For this review, take the finished solid that the model builds, in its own axes (mm). A direction names the side the tool comes from. Coordinates: 2 decimals unless noted, no trailing zeros. Loops run counter-clockwise (first coordinate to the right, second up) from the corner with the lowest first, then second, coordinate; pieces in that order, holes last.
1. Take a section at C-C, the plane x = 0. State the section outline as (y, z) points, then the cut area to 3 significant figures.
2. Take a section at A-A, the plane x = -37.5. State the section outline as (y, z) points, then the cut area to 3 significant figures.
3. To check wall thickness, follow probe 1 along X at (y, z) = (-35.5, 16.5); probe 2 along X at (y, z) = (-24.5, 31); probe 3 along X at (y, z) = (-34, 9). State the ranges of each line that lie inside material, in increasing order.
4. Mouldability with a two-part tool opening along Y and no side actions: class faces 1 (the face through (17, -38, 52.7)), 2 (the face through (-15.788, -17.696, 3.131)), 3 (the face through (17.49, -34.27, 13.36)), 4 (the face through (-39.359, -26.527, 29.569)) as pulls with the +Y half, pulls with the -Y half, needs draft (parallel to the pull), parting line crosses it, or undercut.
5. Take a section at D-D, the plane x = -15.5. State the section outline as (y, z) points, then the cut area to 3 significant figures.
6. Take a section at B-B, the plane y = -24.5. State the section outline as (x, z) points, then the cut area to 3 significant figures.
7. Machinability: for faces 5 (the face through (21.004, -10, 14)), 6 (the face through (15, -34.5, 40)), 7 (the face through (17, -40.85, 39)), 8 (the face through (-7, -27.5, 17)), which of the approach directions +Z, -Z, +X, -X, +Y, -Y give a long, thin tool a straight path to every point of the face, cutting with its end or side? Answer none if there is none.
8. Clearance check with flat-ended pins moving along their axes: P1, Ø6, axis at x = 9.5, z = 25.5, coming from the -Y side; P2, Ø5, axis at x = -21, y = -9, coming from the +Z side; P3, Ø1.5, axis at y = -13, z = 13, coming from the -X side. State where each tip first meets the part, or that it passes through.
Autodesk Inventor part; units mm, degrees
ref_plane "Work Plane1" through (0, -21.15, 0) normal (-1, 0, 0) x (0, 0, 1)
ref_plane "Work Plane2" through (-27.5, -34.5, 33.95) normal (0, -1, 0) x (1, 0, 0)
ref_plane "Work Plane3" through (-33.9, -14.5, 32.7) normal (0, 0, -1) x (0, 1, 0)
sketch "Sketch1" plane through (0, 0, 0) normal (0, 0, 1) x (1, 0, 0)
  line L0 (-21.15, 16.8267) -> (-21.15, -16.8267)
  arc A0 (-21.15, -16.8267) -> (-21.0036, -17.1802) centre (-20.65, -16.8267) ccw
  line L1 (-21.0036, -17.1802) -> (-17.1802, -21.0036)
  arc A1 (-17.1802, -21.0036) -> (-16.8267, -21.15) centre (-16.8267, -20.65) ccw
  line L2 (-16.8267, -21.15) -> (16.8267, -21.15)
  arc A2 (16.8267, -21.15) -> (17.1802, -21.0036) centre (16.8267, -20.65) ccw
  line L3 (17.1802, -21.0036) -> (21.0036, -17.1802)
  arc A3 (21.0036, -17.1802) -> (21.15, -16.8267) centre (20.65, -16.8267) ccw
  line L4 (21.15, -16.8267) -> (21.15, 16.8267)
  arc A4 (21.15, 16.8267) -> (21.0036, 17.1802) centre (20.65, 16.8267) ccw
  line L5 (21.0036, 17.1802) -> (17.1802, 21.0036)
  arc A5 (17.1802, 21.0036) -> (16.8267, 21.15) centre (16.8267, 20.65) ccw
  line L6 (16.8267, 21.15) -> (-16.8267, 21.15)
  arc A6 (-16.8267, 21.15) -> (-17.1802, 21.0036) centre (-16.8267, 20.65) ccw
  line L7 (-17.1802, 21.0036) -> (-21.0036, 17.1802)
  arc A7 (-21.0036, 17.1802) -> (-21.15, 16.8267) centre (-20.65, 16.8267) ccw
  circle A8 centre (-15.5, -15.5) radius 1.75
  circle A9 centre (-15.5, 15.5) radius 1.75
  circle A10 centre (15.5, 15.5) radius 1.75
  circle A11 centre (15.5, -15.5) radius 1.75
  circle A12 centre (0, 0) radius 17
  circle A13 centre (15.5, 15.5) radius 2.2144
  circle A14 centre (15.5, -15.5) radius 2.2144
  circle A15 centre (-15.5, -15.5) radius 2.2144
  circle A16 centre (-15.5, 15.5) radius 2.2144
  circle A17 centre (0, 0) radius 17.7962
extrude "Extrusion1" add sketch "Sketch1" along normal blind 6.35 contours A7 L7 A6 L6 A5 L5 A4 L4 A3 L3 A2 L2 A1 L1 A0 L0
sketch "Sketch2" plane through (-16.8267, -21.15, 0) normal (0, -1, 0) x (1, 0, 0)
  line L0 (0, 0) -> (33.6533, 0)
  line L1 (33.6533, 0) -> (33.6533, 6.35)
  line L2 (0, 6.35) -> (33.6533, 6.35)
  line L3 (0, 0) -> (0, 6.35)
  line L4 (-10.6733, 32.7) -> (65.5267, 32.7)
  line L5 (65.5267, 33.95) -> (-10.6733, 33.95)
  line L6 (65.5267, 33.95) -> (65.5267, 39.1)
  line L7 (65.5267, 39.1) -> (-10.6733, 39.1)
  line L8 (-10.6733, 33.95) -> (-10.6733, 39.1)
  line L9 (0, 0) -> (33.6533, 0)
  line L10 (33.6533, 0) -> (33.6533, 32.7)
  line L11 (33.6533, 32.7) -> (0, 32.7)
  line L12 (0, 32.7) -> (0, 0)
  line L13 (-4.1769, 0) -> (-0.3536, 0)
  line L14 (-0.3536, 0) -> (-0.3536, 6.35)
  line L15 (-4.1769, 6.35) -> (-0.3536, 6.35)
  line L16 (-4.1769, 0) -> (-4.1769, 6.35)
  line L17 (34.0069, 0) -> (37.8302, 0)
  line L18 (37.8302, 0) -> (37.8302, 6.35)
  line L19 (34.0069, 6.35) -> (37.8302, 6.35)
  line L20 (34.0069, 0) -> (34.0069, 6.35)
  line L21 (-4.1769, 0) -> (37.8302, 0)
  line L22 (37.8302, 0) -> (37.8302, 32.7)
  line L23 (37.8302, 32.7) -> (-4.1769, 32.7)
  line L24 (-4.1769, 32.7) -> (-4.1769, 0)
  point P0 (16.8267, 0)
extrude "Extrusion2" add sketch "Sketch2" along normal blind 6.35 contours L3 L2 L1 L0 | L21 L14 L15 L24 L4 L12 L3 | L1 L10 L4 L22 L19 L20 L21 | L12 L4 L10 L2 | L13 L16 L15 L14 | L20 L19 L18 L17
ref_plane "Work Plane1" through (0, -21.15, 0) normal (-1, 0, 0) x (0, 0, 1)
sketch "Sketch4" plane through (-21.0036, -21.15, 0) normal (-1, 0, 0) x (0, 0, 1)
  line L0 (0, 37.9767) -> (0, 4.3233)
  line L1 (0, 4.3233) -> (6.35, 4.3233)
  line L2 (6.35, 37.9767) -> (6.35, 4.3233)
  line L3 (0, 37.9767) -> (6.35, 37.9767)
  line L4 (32.7, 0) -> (0, 0)
  line L5 (0, 0) -> (0, -6.35)
  line L6 (32.7, -6.35) -> (0, -6.35)
  line L7 (32.7, 0) -> (32.7, -6.35)
  line L8 (6.35, 37.9767) -> (6.35, 4.3233)
  line L9 (32.7, 0) -> (32.7, -6.35)
  line L10 (0, 0.1464) -> (6.35, 0.1464)
  line L11 (0, 38.3302) -> (6.35, 38.3302)
  line L12 (0, 38.3302) -> (6.35, 38.3302)
  line L13 (6.35, 38.9462) -> (6.35, 3.3538)
  line L14 (6.35, 38.3302) -> (32.7, 0)
  line L15 (0, 0) -> (0, -6.35)
  line L16 (32.7, 0) -> (0, 0)
  line L17 (0, 0) -> (0, 38.3302)
  point P0 (0, 21.15)
extrude "Extrusion3" add sketch "Sketch4" along normal blind 6.35
mirror "Mirror1" about plane through (0, -21.15, 0) normal (-1, 0, 0) of "Extrusion3"
sketch "Sketch5" plane through (-16.8267, -27.5, 0) normal (0, -1, 0) x (1, 0, 0)
  line L0 (2.5767, 45.45) -> (8.0767, 45.45)
  arc A0 (8.0767, 39.95) -> (8.0767, 45.45) centre (8.0767, 42.7) ccw
  line L1 (8.0767, 39.95) -> (2.5767, 39.95)
  arc A1 (2.5767, 45.45) -> (2.5767, 39.95) centre (2.5767, 42.7) ccw
  line L2 (17.3267, 50.7) -> (-6.6733, 50.7)
  line L3 (-6.6733, 50.7) -> (-6.6733, 34.7)
  line L4 (-6.6733, 34.7) -> (17.3267, 34.7)
  line L5 (17.3267, 34.7) -> (17.3267, 50.7)
  line L6 (-10.5269, 32.7) -> (44.1802, 32.7)
  line L7 (-10.5269, 0) -> (-10.5269, 32.7)
  line L8 (44.1802, 0) -> (-10.5269, 0)
  line L9 (44.1802, 0) -> (44.1802, 32.7)
  line L10 (37.8302, 32.7) -> (44.1802, 32.7)
  line L11 (44.1802, 32.7) -> (24.1802, 32.7)
  line L12 (24.1802, 32.7) -> (24.1802, 26.35)
  line L13 (24.1802, 26.35) -> (44.1802, 26.35)
  line L14 (44.1802, 26.35) -> (44.1802, 32.7)
  point P0 (16.8267, 0)
  dimension "d6" = 20
  dimension "d7" = 6.35
ref_plane "Work Plane2" through (-27.5, -34.5, 33.95) normal (0, -1, 0) x (1, 0, 0)
extrude "Extrusion4" add sketch "Sketch5" along normal up to surface (7 mm away) contours L6 L9 L13 L12
sketch "Sketch6" plane through (7.3536, -34.5, 32.7) normal (0, -1, 0) x (1, 0, 0)
  line L0 (20, 0) -> (20, -6.35)
  line L1 (0, 0) -> (20, 0)
  line L2 (0, -6.35) -> (0, 0)
  line L3 (20, -6.35) -> (0, -6.35)
  point P0 (-7.3536, -32.7)
extrude "Extrusion5" add sketch "Sketch6" along normal blind 6.35
sketch "Sketch7" plane through (-27.3536, -21.15, 32.7) normal (0, 0, 1) x (1, 0, 0)
  line L0 (34.7071, -6.35) -> (34.7071, -19.7)
  line L1 (54.7071, 0) -> (54.7071, -19.7)
  line L2 (34.7071, -19.7) -> (54.7071, -19.7)
  line L3 (54.7071, -19.7) -> (54.7071, -13.35)
  line L4 (54.7071, -13.35) -> (34.7071, -13.35)
  line L5 (34.7071, -13.35) -> (34.7071, -19.7)
  point P0 (27.3536, 21.15)
  dimension "d12" = 6.35
extrude "Extrusion6" add sketch "Sketch7" along normal blind 20
sketch "Sketch8" plane through (7.3536, -40.85, 32.7) normal (0, -1, 0) x (1, 0, 0)
  line L0 (20, 20) -> (0, 20)
  line L1 (20, -6.35) -> (20, 20)
  line L2 (0, 20) -> (20, 20)
  line L3 (20, 20) -> (20, 0)
  line L4 (20, 0) -> (0, 0)
  line L5 (0, 0) -> (0, 20)
  circle A0 centre (10, 10) radius 2.75
  point P0 (-7.3536, -32.7)
  dimension "d15" = 20
  dimension "d16" = 5.5
extrude "Extrusion7" cut sketch "Sketch8" against normal blind 20 contours A0
ref_plane "Work Plane3" through (-33.9, -14.5, 32.7) normal (0, 0, -1) x (0, 1, 0)
sketch "Sketch9" plane through (-33.9, -14.5, 32.7) normal (0, 0, -1) x (0, 1, 0)
  line L0 (0, -12.35) -> (-1000, -12.35)
  line L1 (0, -12.35) -> (0, -7.2)
  line L2 (0, -7.2) -> (-1000, -7.2) construction
  line L3 (-1000, -12.35) -> (-1000, -7.2)
  line L4 (-1000, 5.15) -> (0, 5.15) construction
  line L5 (-1000, 0) -> (-1000, 5.15)
  line L6 (0, 0) -> (-1000, 0) construction
  line L7 (0, 0) -> (0, 5.15)
  line L8 (0, 5.15) -> (-40, 5.15) construction
  line L9 (-40, 5.15) -> (-40, -12.35)
  line L10 (-40, -12.35) -> (0, -12.35)
  line L11 (0, -12.35) -> (0, 5.15)
  line L12 (-6.5036, 51.0802) -> (-2.6802, 54.9036)
  arc A0 (-6.5036, 51.0802) -> (-6.65, 50.7267) centre (-6.15, 50.7267) ccw
  line L13 (-6.65, 50.7267) -> (-6.65, 54.9036)
  line L14 (-2.6802, 54.9036) -> (-6.65, 54.9036)
  line L15 (31.6802, 54.9036) -> (31.6802, 61.2536)
  line L16 (31.6802, 61.2536) -> (-13, 61.2536)
  line L17 (-13, 61.2536) -> (-13, 6.5464)
  line L18 (31.6802, 6.5464) -> (-13, 6.5464)
  line L19 (31.6802, 12.8964) -> (31.6802, 6.5464)
  line L20 (35.5036, 16.7198) -> (31.6802, 12.8964)
  arc A1 (35.5036, 16.7198) -> (35.65, 17.0733) centre (35.15, 17.0733) ccw
  line L21 (35.65, 50.7267) -> (35.65, 17.0733)
  arc A2 (35.65, 50.7267) -> (35.5036, 51.0802) centre (35.15, 50.7267) ccw
  line L22 (31.6802, 54.9036) -> (35.5036, 51.0802)
  line L23 (-6.65, 12.8964) -> (-6.65, 17.0733)
  arc A3 (-6.65, 17.0733) -> (-6.5036, 16.7198) centre (-6.15, 17.0733) ccw
  line L24 (-2.6802, 12.8964) -> (-6.5036, 16.7198)
  line L25 (-2.6802, 12.8964) -> (-6.65, 12.8964)
  circle A4 centre (14.5, 33.9) radius 17.7962
  circle A5 centre (30, 18.4) radius 2.2144
  circle A6 centre (-1, 18.4) radius 2.2144
  circle A7 centre (-1, 49.4) radius 2.2144
  circle A8 centre (30, 49.4) radius 2.2144
  line L26 (0, 5.15) -> (-40, 5.15) construction
  line L27 (-40, 5.15) -> (-40, 6.5464)
  line L28 (-40, 6.5464) -> (0, 6.5464)
  line L29 (0, 6.5464) -> (0, 5.15)
  line L30 (-20, -3.6) -> (-40, -3.6) construction
  line L31 (-20, -12.35) -> (-20, 6.5464) construction
  line L32 (-20, -3.6) -> (0, -3.6) construction
  circle A9 centre (-10, -3.6) radius 2.75
  circle A10 centre (-30, -3.6) radius 2.75
  line L33 (0, -12.35) -> (-40, -12.35)
  line L34 (-40, -12.35) -> (-40, 6.5464)
  line L35 (-40, 6.5464) -> (0, 6.5464)
  line L36 (0, 6.5464) -> (0, -12.35)
  dimension "d19" = 40
  dimension "d20" = 5.5
extrude "Extrusion8" add sketch "Sketch9" along normal blind 6.35 contours L0 L9 L27 L28 L18 L29 L7 L11 L1
sketch "Sketch10" plane through (-27.3536, -54.5, 32.7) normal (1, 0, 0) x (0, 0, -1)
  line L0 (-1.6, 40) -> (-1.6, -960)
  line L1 (6.35, 27) -> (0, 27)
  line L2 (0, 27) -> (0, 0)
  line L3 (0, 0) -> (6.35, 0)
  line L4 (6.35, 27) -> (6.35, 0)
  point P0 (32.7, 54.5)
extrude "Extrusion9" add sketch "Sketch10" along normal blind 6.35
sketch "Sketch11" plane through (-21.0036, -54.5, 32.7) normal (1, 0, 0) x (0, 0, -1)
  line L0 (0, 27) -> (6.35, 27)
  line L1 (0, 27) -> (0, 0)
  line L2 (0, 0) -> (6.35, 0)
  line L3 (6.35, 0) -> (6.35, 27)
  line L4 (32.7, 27) -> (6.35, 27)
  line L5 (0, 0) -> (6.35, 0)
  line L6 (32.7, 27) -> (6.35, 0)
  line L7 (6.35, 27) -> (6.35, 13.65)
  line L8 (6.35, 0) -> (6.35, 27)
  line L9 (32.7, 71.6802) -> (32.7, 27)
  line L10 (6.35, 27) -> (32.7, 27)
  point P0 (32.7, 54.5)
extrude "Extrusion10" add sketch "Sketch11" against normal blind 6.35 contours L4 L6 L3
sketch "Sketch12" plane through (-27.3536, -21.15, 32.7) normal (1, 0, 0) x (0, 0, -1)
  line L0 (0, 0) -> (4.5715, 6.65)
  line L1 (0, 6.65) -> (4.5715, 6.65)
  line L2 (0, 6.65) -> (0, 0)
  point P0 (32.7, 21.15)
extrude "Extrusion11" add sketch "Sketch12" along normal up to surface (6.35 mm away)
sketch "Sketch13" plane through (27.3536, -27.5, 0) normal (1, 0, 0) x (0, 0, -1)
  line L0 (0, 44.6802) -> (0, 0)
  line L1 (-6.35, 44.6802) -> (0, 44.6802)
  line L2 (-32.7, 6.35) -> (-6.35, 44.6802)
  line L3 (-32.7, 6.35) -> (-32.7, -7)
  line L4 (-32.7, -7) -> (-52.7, -7)
  line L5 (-52.7, -13.35) -> (-52.7, -7)
  line L6 (-26.35, -13.35) -> (-52.7, -13.35)
  line L7 (-26.35, 0) -> (-26.35, -13.35)
  line L8 (0, 0) -> (-26.35, 0)
  line L9 (-26.35, -13.35) -> (0, 0)
  line L10 (-26.35, 0) -> (-26.35, -13.35)
  line L11 (-26.35, 13) -> (-26.35, -27)
  line L12 (-32.7, 0) -> (0, 0)
  line L13 (-26.35, 0) -> (0, 0)
  point P0 (0, 27.5)
extrude "Extrusion12" add sketch "Sketch13" against normal up to surface (20 mm away) contours L9 L7 L8
sketch "Sketch14" plane through (0, 0, 0) normal (0, 0, -1) x (-1, 0, 0)
  line L0 (-17.1802, -21.0036) -> (-21.0036, -17.1802)
  arc A0 (-17.1802, -21.0036) -> (-16.8267, -21.15) centre (-16.8267, -20.65) ccw
  line L1 (-16.8267, -21.15) -> (-21.0036, -21.15)
  line L2 (-21.0036, -17.1802) -> (-21.0036, -21.15)
  line L3 (-21.0036, 17.1802) -> (-27.3536, 17.1802)
  line L4 (-27.3536, 17.1802) -> (-27.3536, -27.5)
  line L5 (-27.3536, -27.5) -> (-7.3536, -27.5)
  line L6 (-7.3536, -27.5) -> (21.0036, -27.5)
  line L7 (21.0036, -27.5) -> (27.3536, -27.5)
  line L8 (27.3536, 17.1802) -> (27.3536, -27.5)
  line L9 (21.0036, 17.1802) -> (27.3536, 17.1802)
  line L10 (17.1802, 21.0036) -> (21.0036, 17.1802)
  arc A1 (17.1802, 21.0036) -> (16.8267, 21.15) centre (16.8267, 20.65) ccw
  line L11 (-16.8267, 21.15) -> (16.8267, 21.15)
  arc A2 (-16.8267, 21.15) -> (-17.1802, 21.0036) centre (-16.8267, 20.65) ccw
  line L12 (-21.0036, 17.1802) -> (-17.1802, 21.0036)
  line L13 (21.0036, -21.15) -> (16.8267, -21.15)
  arc A3 (16.8267, -21.15) -> (17.1802, -21.0036) centre (16.8267, -20.65) ccw
  line L14 (21.0036, -17.1802) -> (17.1802, -21.0036)
  line L15 (21.0036, -17.1802) -> (21.0036, -21.15)
  circle A4 centre (0, 0) radius 17.7962
  circle A5 centre (15.5, 15.5) radius 2.2144
  circle A6 centre (15.5, -15.5) radius 2.2144
  circle A7 centre (-15.5, -15.5) radius 2.2144
  circle A8 centre (-15.5, 15.5) radius 2.2144
extrude "Extrusion13" add sketch "Sketch14" against normal up to surface (6.35 mm away) contours A0 L1 L2 L0 | L13 A3 L14 L15
properties part number "motorBracket"
Results list:
1. outline: (-27.5, 0) - (-17.8, 0) - (-17.8, 6.35) - (-21.15, 6.35) - (-21.15, 32.7) - (-27.5, 32.7) - close; (17.8, 0) - (21.15, 0) - (21.15, 6.35) - (17.8, 6.35) - close
1. area: 250 mm2
2. outline: (-54.5, 26.35) - (-47.25, 26.35) - (-47.25, 32.7) - (-54.5, 32.7) - close; (-41.75, 26.35) - (-27.25, 26.35) - (-27.25, 32.7) - (-41.75, 32.7) - close; (-21.75, 26.35) - (-14.5, 26.35) - (-14.5, 32.7) - (-21.75, 32.7) - close
2. area: 184 mm2
3. probe 1: x = -27.35 to -21, 7.35 to 27.35
3. probe 2: x = -46.25 to -40.25, -34.75 to 27.35
3. probe 3: x = -27.35 to -21
4. face 1: needs draft
4. face 2: undercut
4. face 3: pulls with the -Y half
4. face 4: undercut
5. outline: (-27.5, 0) - (-17.71, 0) - (-17.71, 6.35) - (-21.15, 6.35) - (-21.15, 32.7) - (-27.5, 32.7) - close; (-13.29, 0) - (-8.74, 0) - (-8.74, 6.35) - (-13.29, 6.35) - close; (8.74, 0) - (13.29, 0) - (13.29, 6.35) - (8.74, 6.35) - close; (17.71, 0) - (21.15, 0) - (21.15, 6.35) - (17.71, 6.35) - close
5. area: 309 mm2
6. outline: (-46.25, 26.35) - (-40.25, 26.35) - (-40.25, 32.7) - (-46.25, 32.7) - close; (-34.75, 26.35) - (-27.35, 26.35) - (-27.35, 0) - (27.35, 0) - (27.35, 32.7) - (-34.75, 32.7) - close
6. area: 1,870 mm2
7. face 5: +Z, +Y
7. face 6: +Z, +X, -X, +Y
7. face 7: +Z, -Z, +X, -Y
7. face 8: +Z, -Z, -Y
8. P1: stops at y = -40.85
8. P2: stops at z = 26.07
8. P3: stops at x = -27.35
